Geometry: see drawing. Coordinates: mm, zero at the bounding-box minimum. A direction names the side the tool comes from. Coordinates: 2 decimals unless noted, no trailing zeros. Loops run counter-clockwise (first coordinate to the right, second up) from the corner with the lowest first, then second, coordinate; pieces in that order, holes last. Notation, with made-up numbers: (30.25, -36) -> (75.25, -36) arc R20 ccw to (75.25, -12) -> close; hole circle Ø4 at (-31.75, 14.5). An arc over 180 degrees is marked (long way). One line per item, written item: value. Start each with the question number.
Item 1: Section query A-A on y = 8. Return loops of the section in (x, z), then the cut area to 3 significant figures.
Item 2: Ray query, probe 1 along Z at (x, y) = (34.5, 0.7); probe 2 along Y at (x, z) = (24.5, 2); probe 3 along Y at (x, z) = (29, 1.6). Return the intervals inside material, ascending. Write a range as from..to.
Item 3: Section query C-C on x = 34.5. Return loops of the section in (y, z), then the cut area to 3 significant figures.
Item 4: Contact query for flat-ended pins moving along their axis: pin 1 Ø1.6 at (x, z) = (24, 1.5) entering from -Y; pin 2 Ø8.5 at (x, z) = (19, 10.5) entering from +Y; pin 3 Ø1.5 at (x, y) = (19.5, 10.5) entering from +Z; pin 4 Ø2.5 at (x, z) = (4.5, 7.5) entering from +Y. Output: stop coordinate, or through.
Item 5: Section query B-B on z = 7.5. Return loops of the section in (x, y), then the cut area to 3 significant figures.
Item 6: Set-up query: the marked faces 1 and 2. Return all of +Z, -Z, +X, -X, +Y, -Y with unobstructed straight access to the full face (end or side cutting, diameter ignored); none if empty.
Item 7: Section query D-D on x = 21. Return loops of the section in (y, z), then the cut area to 3 significant figures.
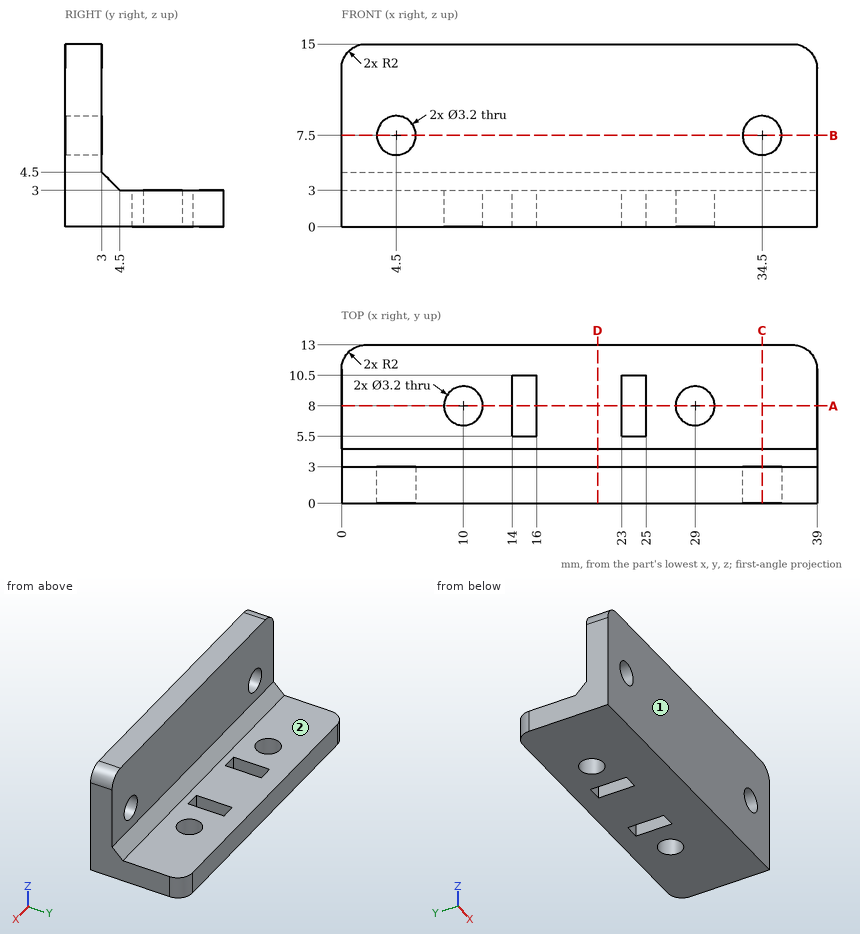
Reply:
1. outline: (0, 0) -> (8.4, 0) -> (8.4, 3) -> (0, 3) -> close; (11.6, 0) -> (14, 0) -> (14, 3) -> (11.6, 3) -> close; (16, 0) -> (23, 0) -> (23, 3) -> (16, 3) -> close; (25, 0) -> (27.4, 0) -> (27.4, 3) -> (25, 3) -> close; (30.6, 0) -> (39, 0) -> (39, 3) -> (30.6, 3) -> close
1. area: 85.8 mm²
2. probe 1: z = 0..5.9, 9.1..15
2. probe 2: y = 0..5.5, 10.5..13
2. probe 3: y = 0..6.4, 9.6..13
3. outline: (0, 0) -> (13, 0) -> (13, 3) -> (4.5, 3) -> (3, 4.5) -> (3, 5.9) -> (0, 5.9) -> close; (0, 9.1) -> (3, 9.1) -> (3, 15) -> (0, 15) -> close
3. area: 66.5 mm²
4. pin 1: stops at y = 0
4. pin 2: stops at y = 3
4. pin 3: stops at z = 3
4. pin 4: passes through
5. outline: (0, 0) -> (2.9, 0) -> (2.9, 3) -> (0, 3) -> close; (6.1, 0) -> (32.9, 0) -> (32.9, 3) -> (6.1, 3) -> close; (36.1, 0) -> (39, 0) -> (39, 3) -> (36.1, 3) -> close
5. area: 97.8 mm²
6. face 1: +Z, -Z, +X, -X, -Y
6. face 2: +Z, +X, -X, +Y
7. outline: (0, 0) -> (13, 0) -> (13, 3) -> (4.5, 3) -> (3, 4.5) -> (3, 15) -> (0, 15) -> close
7. area: 76.1 mm²
